Design review of the part built by this model. Coordinates are the model's own, in mm. A direction names the side the tool comes from. Coordinates: 2 decimals unless noted, no trailing zeros. Loops run counter-clockwise (first coordinate to the right, second up) from the corner with the lowest first, then second, coordinate; pieces in that order, holes last.
Q1. Wall thickness on probe 1 along Y at (x, z) = (-7.75, 0); probe 2 along X at (y, z) = (6, 0); probe 3 along Y at (x, z) = (10.5, 11.5): over which ranges is each line inside the solid? List them lowest first.
Q2. Add section C-C on z = 5.5. Give the boundary of the cut face in (x, y).
Q3. For P1, Ø3, axis at x = 17.5, y = 7, coming from the +Z side; P2, Ø2.5, axis at y = 5, z = 0, coming from the -X side; P3, Ø2, axis at x = 7, z = 11, coming from the +Y side, all flat-tipped, find the tip position at first contact; note any pin that passes through.
Q4. Add section A-A on z = 0. Give the boundary of the cut face in (x, y), and give its area (3 significant figures).
Q5. Add section B-B on x = 5.5. Give the boundary of the cut face in (y, z), and give its area (3 significant figures).
Q6. Add section D-D on y = 9. Give the boundary of the cut face in (x, z), and give its area (3 significant figures).
Q7. Draft analysis for pull direction Z (two halves, no side actions). For faces 1 (the face through (6.057, 4.93, -1.907)), 2 (the face through (25.76, 2, 0)), 3 (the face through (23.55, 2.46, 16.65)), 4 (the face through (-7.75, 3.76, -0.65)), state which applies: released by +Z, released by -Z, zero draft, split by the parting line, or undercut.
Q8. Machinability: for faces 5 (the face through (12, 0, 0)), 6 (the face through (-9.34, 7.15, -0.41)), which of the approach directions +Z, -Z, +X, -X, +Y, -Y give a long, thin tool a straight path to every point of the face, cutting with its end or side? Answer none if there is none.
```python
from build123d import *

# Parameters (mm, degrees)
SKETCH1_R           = 9.35
SKETCH1_R_2         = 6.35
SKETCH1_R_3         = 5
BOSS_EXTRUDE1_DEPTH = 5
SKETCH1_3_R         = 9.35
SKETCH1_3_R_2       = 6.35
BOSS_EXTRUDE2_DEPTH = 10
SKETCH2_R           = 1.4
CUT_EXTRUDE1_DEPTH  = 10.35


with BuildPart() as part:
    # Sketch1 → Boss-Extrude1 (new body)
    with BuildSketch(Plane(origin=(0, 0, 0), x_dir=(1, 0, 0), z_dir=(0, 1, 0))):
        Circle(SKETCH1_R)
        Circle(SKETCH1_R_2, mode=Mode.SUBTRACT)
        with BuildLine():
            Line((18.991661947, 17.176855838), (-3.306792159, 8.745720417))
            ThreePointArc((-3.306792159, 8.745720417), (5.315260733, 7.692236563), (9.35, 0))
            ThreePointArc((9.35, 0), (5.315260733, -7.692236563), (-3.306792159, -8.745720417))
            Line((-3.306792159, -8.745720417), (18.991661947, -17.176855838))
            ThreePointArc((18.991661947, -17.176855838), (17.917614581, -8.386504512), (25.76, -12.5))
            Line((25.76, -12.5), (25.76, 12.5))
            ThreePointArc((25.76, 12.5), (17.917614581, 8.386504512), (18.991661947, 17.176855838))
        make_face()
        with Locations((20.76, 12.5)):
            Circle(SKETCH1_R_3)
        with Locations((20.76, -12.5)):
            Circle(SKETCH1_R_3)
    extrude(amount=BOSS_EXTRUDE1_DEPTH)

    # Sketch1_3 → Boss-Extrude2 (add)
    with BuildSketch(Plane(origin=(0, 0, 0), x_dir=(1, 0, 0), z_dir=(0, 1, 0))):
        Circle(SKETCH1_3_R)
        Circle(SKETCH1_3_R_2, mode=Mode.SUBTRACT)
    extrude(amount=BOSS_EXTRUDE2_DEPTH)

    # Sketch2 → Cut-Extrude1 (cut, through all)
    with BuildSketch(Plane(origin=(0, 0, 0), x_dir=(0, 0, -1), z_dir=(1, 0, 0))):
        with Locations((0, 5)):
            Circle(SKETCH2_R)
    extrude(amount=-CUT_EXTRUDE1_DEPTH, mode=Mode.SUBTRACT)


solid = part.part
```
Entries:
1. probe 1: y = 0 to 3.6, 6.4 to 10
1. probe 2: x = 6.35 to 9.35
1. probe 3: y = 0 to 5
2. outline: (-7.56, 0) - (-3.17, 0) - (-3.17, 10) - (-7.56, 10) - close; (3.17, 0) - (25.76, 0) - (25.76, 5) - (7.56, 5) - (7.56, 10) - (3.17, 10) - close
3. P1: passes through
3. P2: stops at x = 6.23
3. P3: stops at y = 5
4. outline: (-9.35, 0) - (-6.35, 0) - (-6.35, 3.6) - (-9.35, 3.6) - close; (-9.35, 6.4) - (-6.35, 6.4) - (-6.35, 10) - (-9.35, 10) - close; (6.35, 0) - (25.76, 0) - (25.76, 5) - (9.35, 5) - (9.35, 10) - (6.35, 10) - close
4. area: 134 mm2
5. outline: (0, -12.08) - (5, -12.08) - (5, -7.56) - (10, -7.56) - (10, -3.17) - (0, -3.17) - close; (0, 3.17) - (10, 3.17) - (10, 7.56) - (5, 7.56) - (5, 12.08) - (0, 12.08) - close
5. area: 133 mm2
6. outline: circle Ø18.7 at (0, 0); hole circle Ø12.7 at (0, 0)
6. area: 148 mm2
7. face 1: undercut
7. face 2: zero draft
7. face 3: released by +Z
7. face 4: undercut
8. face 5: +Z, -Z, +X, -X, -Y
8. face 6: +Y
